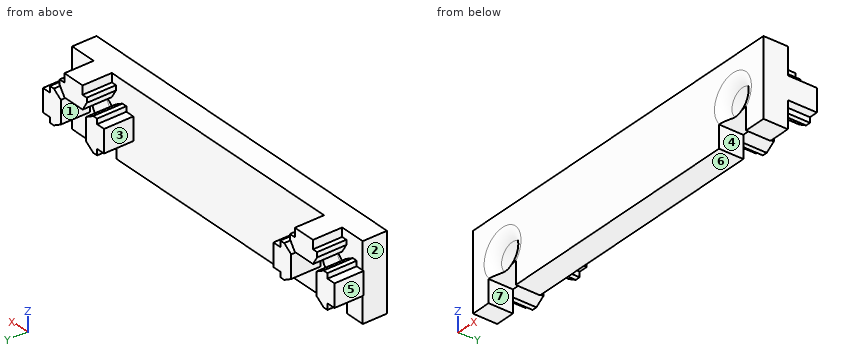
```python
from build123d import *

# Parameters (mm, degrees)
BOSS_EXTRUDE1_DEPTH   = 7.62
BOSS_EXTRUDE1_2_DEPTH = 7.62
BOSS_EXTRUDE1_3_DEPTH = 7.62
BOSS_EXTRUDE1_4_DEPTH = 7.62
SKETCH2_W             = 132.9538108
SKETCH2_H             = 20
BOSS_EXTRUDE2_DEPTH   = 6.35
LPATTERN2_COUNT       = 2
LPATTERN2_PITCH       = 75.4126
CUT_EXTRUDE1_DEPTH    = 125.148300392
FILLET1_R             = 2.54
SKETCH13_R            = 3.5
CUT_EXTRUDE5_DEPTH    = 124.59491895
FILLET6_R             = 2.54
SKETCH14_W            = 8.89
SKETCH14_H            = 5.842
CUT_EXTRUDE6_DEPTH    = 125.148300392
SKETCH15_W            = 25.4
SKETCH15_H            = 40.894
BOSS_EXTRUDE3_DEPTH   = 12.7
FILLET15_R            = 10.16
FILLET16_R            = 10.16
FILLET17_R            = 10.16
FILLET18_R            = 10.16
SKETCH18_R            = 1.984375
CUT_EXTRUDE9_DEPTH    = 12.7
SKETCH19_W            = 37.866917971
SKETCH19_H            = 35.1892
CUT_EXTRUDE10_DEPTH   = 133.001722138


with BuildPart() as part:
    # Sketch1 → Boss-Extrude1 (new body)
    with BuildSketch(Plane(origin=(0, 0, 0), x_dir=(1, 0, 0), z_dir=(0, 1, 0))):
        Polygon((2.9718, 10), (-2.9718, 10), (-2.9718, 7.714), (-4.567901235, 7.714), (-4.567901235, 6.444), (-2.9718, 4.158), (2.9718, 4.158), (4.322098765, 6.444), (4.322098765, 7.714), (2.9718, 7.714), align=None)
    boss_extrude1 = extrude(amount=BOSS_EXTRUDE1_DEPTH)



with BuildPart() as body_2:
    # Sketch1 → Boss-Extrude1 2 (new body)
    with BuildSketch(Plane(origin=(0, 0, 0), x_dir=(1, 0, 0), z_dir=(0, 1, 0))):
        Polygon((4.158, -2.9718), (4.158, 2.9718), (6.444, 4.322098765), (7.714, 4.322098765), (7.714, 2.9718), (10, 2.9718), (10, -2.9718), (7.714, -2.9718), (7.714, -4.567901235), (6.444, -4.567901235), align=None)
    boss_extrude1_2 = extrude(amount=BOSS_EXTRUDE1_2_DEPTH)


with BuildPart() as body_3:
    # Sketch1 → Boss-Extrude1 3 (new body)
    with BuildSketch(Plane(origin=(0, 0, 0), x_dir=(1, 0, 0), z_dir=(0, 1, 0))):
        Polygon((-10, -2.9718), (-10, 2.9718), (-7.714, 2.9718), (-7.714, 4.567901235), (-6.444, 4.567901235), (-4.158, 2.9718), (-4.158, -2.9718), (-6.444, -4.322098765), (-7.714, -4.322098765), (-7.714, -2.9718), align=None)
    boss_extrude1_3 = extrude(amount=BOSS_EXTRUDE1_3_DEPTH)


with BuildPart() as body_4:
    # Sketch1 → Boss-Extrude1 4 (new body)
    with BuildSketch(Plane(origin=(0, 0, 0), x_dir=(1, 0, 0), z_dir=(0, 1, 0))):
        Polygon((4.567901235, -6.444), (2.9718, -4.158), (-2.9718, -4.158), (-4.322098765, -6.444), (-4.322098765, -7.714), (-2.9718, -7.714), (-2.9718, -10), (2.9718, -10), (2.9718, -7.714), (4.567901235, -7.714), align=None)
    boss_extrude1_4 = extrude(amount=BOSS_EXTRUDE1_4_DEPTH)


with BuildPart() as part_1:
    add(part.part)

    add(body_2.part)  # Boss-Extrude2 merges body 2

    add(body_3.part)  # Boss-Extrude2 merges body 3

    add(body_4.part)  # Boss-Extrude2 merges body 4
    # Sketch2 → Boss-Extrude2 (add)
    with BuildSketch(Plane.XZ):
        with Locations((-56.4769054, 0)):
            Rectangle(SKETCH2_W, SKETCH2_H)
    extrude(amount=BOSS_EXTRUDE2_DEPTH)

    # LPattern2: Boss-Extrude1, Boss-Extrude1 2, Boss-Extrude1 3, Boss-Extrude1 4 ×2
    with Locations(*[(-i * LPATTERN2_PITCH, 0, 0) for i in range(1, LPATTERN2_COUNT)]):
        add(boss_extrude1)
        add(boss_extrude1_2)
        add(boss_extrude1_3)
        add(boss_extrude1_4)

    # Sketch4 → Cut-Extrude1 (cut, through all)
    with BuildSketch(Plane(origin=(0, -6.35, 0), x_dir=(-1, 0, 0), z_dir=(0, -1, 0))):
        Polygon((122.9538108, -10), (85.4126108, -10), (122.9538108, -0.2108), align=None)
    extrude(amount=-CUT_EXTRUDE1_DEPTH, mode=Mode.SUBTRACT)

    # Fillet1
    fillet1_edges = [part_1.edges().sort_by_distance(p)[0] for p in [
        (-85.4126108, -3.175, 10),
    ]]
    fillet(fillet1_edges, radius=FILLET1_R)

    # Sketch13 → Cut-Extrude5 (cut, through all)
    with BuildSketch(Plane(origin=(0, 0, 0), x_dir=(1, 0, 0), z_dir=(0, 1, 0))):
        with Locations(Location((0, 0, 0), (0, 0, 270))):
            Circle(SKETCH13_R)
        with Locations(Location((-75.4126, 0, 0), (0, 0, 270))):
            Circle(SKETCH13_R)
    extrude(amount=-CUT_EXTRUDE5_DEPTH, mode=Mode.SUBTRACT)

    # Fillet6
    fillet6_edges = [part_1.edges().sort_by_distance(p)[0] for p in [
        (0, -6.35, -3.5),
        (-75.4126, -6.35, -3.5),
    ]]
    fillet(fillet6_edges, radius=FILLET6_R)

    # Sketch14 → Cut-Extrude6 (cut, through all)
    with BuildSketch(Plane(origin=(0, 7.62, 0), x_dir=(1, 0, 0), z_dir=(0, 1, 0))):
        with Locations((-0.122901235, 7.079)):
            Rectangle(SKETCH14_W, SKETCH14_H)
        with Locations((-75.535501235, 7.079)):
            Rectangle(SKETCH14_W, SKETCH14_H)
    extrude(amount=-CUT_EXTRUDE6_DEPTH, mode=Mode.SUBTRACT)

    # Sketch15 → Boss-Extrude3 (add)
    with BuildSketch(Plane.ZY.offset(122.9538108)):
        with Locations((-12.4892, -20.447)):
            Rectangle(SKETCH15_W, SKETCH15_H)
    extrude(amount=-BOSS_EXTRUDE3_DEPTH)

    # Fillet15
    fillet15_edges = [part_1.edges().sort_by_distance(p)[0] for p in [
        (-110.2538108, -6.35, -4.8946),
    ]]
    fillet(fillet15_edges, radius=FILLET15_R)

    # Fillet16
    fillet16_edges = [part_1.edges().sort_by_distance(p)[0] for p in [
        (-110.2538108, -8.255, -10),
    ]]
    fillet(fillet16_edges, radius=FILLET16_R)

    # Fillet17
    fillet17_edges = [part_1.edges().sort_by_distance(p)[0] for p in [
        (-110.2538108, -40.894, -12.4892),
    ]]
    fillet(fillet17_edges, radius=FILLET17_R)

    # Fillet18
    fillet18_edges = [part_1.edges().sort_by_distance(p)[0] for p in [
        (-107.278015697, -9.325795103, 0.2108),
        (-121.6838108, -40.894, 0.2108),
        (-110.2538108, -23.622, 0.2108),
        (-113.229605903, -37.918204897, 0.2108),
    ]]
    fillet(fillet18_edges, radius=FILLET18_R)

    # Sketch18 → Cut-Extrude9 (cut)
    with BuildSketch(Plane.ZY.offset(122.9538108)):
        with Locations((-12.4892, -28.194)):
            Circle(SKETCH18_R)
    extrude(amount=-CUT_EXTRUDE9_DEPTH, mode=Mode.SUBTRACT)

    # Sketch19 → Cut-Extrude10 (cut, through all)
    with BuildSketch(Plane(origin=(0, 0, 0), x_dir=(1, 0, 0), z_dir=(0, 1, 0))):
        with Locations((-104.020351815, 7.5946)):
            Rectangle(SKETCH19_W, SKETCH19_H)
    extrude(amount=-CUT_EXTRUDE10_DEPTH, mode=Mode.SUBTRACT)


solid = part_1.part
```
Geometry check sheet. Reference: the model listing, model coordinates, mm. Face numbers are marked on the shaded views. A direction names the side the tool comes from. Coordinates: 2 decimals unless noted, no trailing zeros. Order: outer loops, then holes, each group sorted by start corner. A loop starts at its lowest first (then second) coordinate and runs counter-clockwise, first axis right, second up. Notation, with made-up numbers: (57, -8.5) - (111, -8.5) arc R19 cw to (111, 3.5) - close; hole circle Ø11 at (5, -13). An arc over 180 degrees is marked (long way). Answer in a Markdown table with one row per item. Add a question column.
1. Access from +Z, -Z, +X, -X, +Y, -Y to the whole of each face (thin tool, end or side, straight path). Record for the marked faces 1, 2, 3 and 4.
2. Draft check along X on the marked faces 5, 6 and 7. Enter one of: +X half, -X half, draft (parallel to the pull), parting line (faces both ways), or undercut.
3. Material ranges on L1, parallel to X at y = 2.75, z = -2.5; L2, parallel to X at y = -2.45, z = 0; L3, parallel to X at y = -5.5, z = -1, recorded low to high. Write a range as [from, to].
4. Section check A-A (z = 0). Give the number of separate pieces and of enclosed holes in the cut face, plus the area to 3 significant figures.
5. Section check C-C (y = -2.75). Enter the section's corners in (x, z).
6. Section check B-B (x = 0). Enter the section's corners in (y, z).
7. Gauge pin test, flat ends, axial feed: pin 1 Ø1.1 at (y, z) = (5, 9) entering from +X; pin 2 Ø4 at (x, z) = (-55.5, -0.5) entering from +Y; pin 3 Ø6.5 at (x, y) = (1, 4.5) entering from -Z. Record the tip position at first contact, or that the pin passes through.
Data:
| question | item | result |
|---|---|---|
| 1 | face 1 | -Z, +Y |
| 1 | face 2 | +Z, -Z, -X, -Y |
| 1 | face 3 | +Z, -Z, +Y |
| 1 | face 4 | -Z, +Y, -Y |
| 2 | face 5 | -X half |
| 2 | face 6 | draft |
| 2 | face 7 | undercut |
| 3 | L1 | x = [-85.41, -79.57], [-71.25, -65.41], [-10, -4.16], [4.16, 10] |
| 3 | L2 | x = [-85.09, -78.91], [-71.91, -3.5], [3.5, 10] |
| 3 | L3 | x = [-85.09, -79.43], [-71.39, -4.02], [4.02, 10] |
| 4 | separate pieces | 3 |
| 4 | enclosed holes | 0 |
| 4 | area | 687 mm² |
| 5 | outline | (-85.09, -10) - (-79.98, -10) - (-79.98, -4.16) - (-71.09, -4.16) - (-71.09, -10) - (-4.57, -10) - (-4.57, -4.16) - (4.32, -4.16) - (4.32, -10) - (10, -10) - (10, 10) - (-85.09, 10) - close; hole circle Ø7 at (-75.41, 0); hole circle Ø7 at (0, 0) |
| 6 | outline | (-6.35, 6.04) arc R2.54 ccw to (-3.81, 3.5) - (0, 3.5) - (0, 4.16) - (7.62, 4.16) - (7.62, 10) - (-6.35, 10) - close; (-5.52, -4.16) - (0, -4.16) - (0, -3.5) - (-3.81, -3.5) arc R2.54 ccw to start |
| 7 | pin 1 | stops at x = 2.97 |
| 7 | pin 2 | stops at y = 0 |
| 7 | pin 3 | stops at z = -3.03 |
